For this review, use the dimensioned drawing (mm, ordinates from the lowest corner) and the shaded views. Give positions to 0.01 mm unless a question says otherwise; leave off trailing zeros. Order: outer loops, then holes, each group sorted by start corner. A loop starts at its lowest first (then second) coordinate and runs counter-clockwise, first axis right, second up.
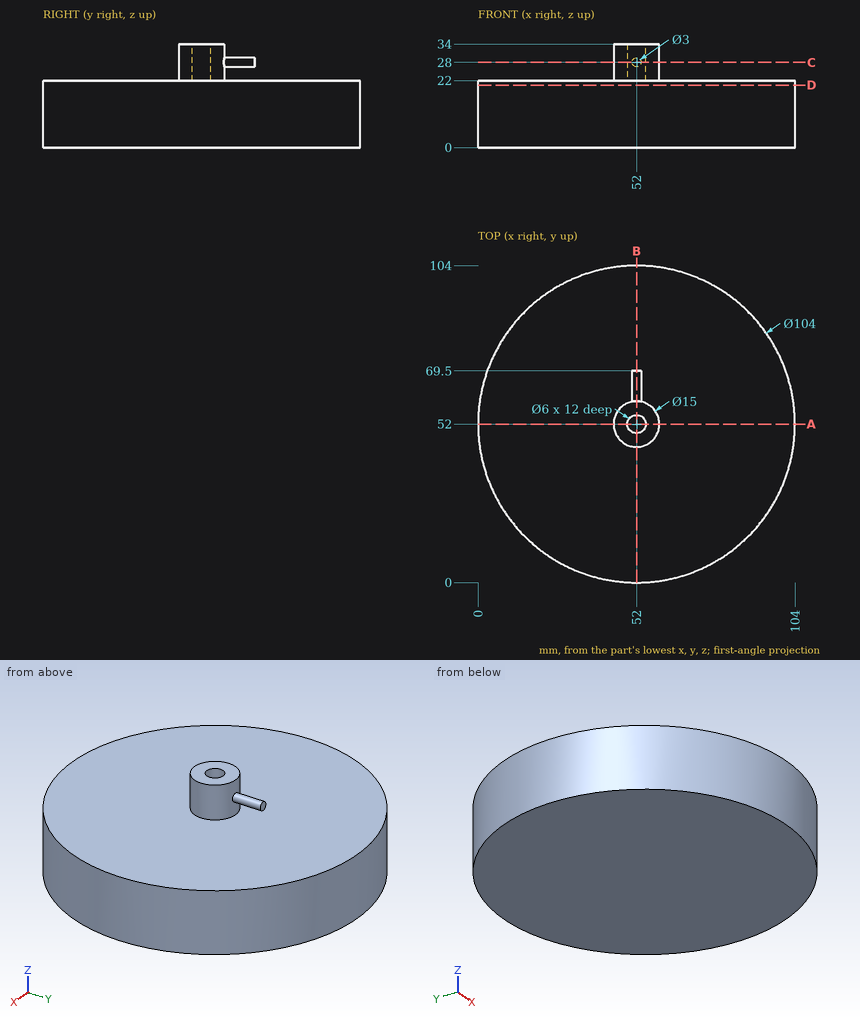
1. For line 1 along Y through (x, z) = (52, 24.5); line 2 along Z through (x, y) = (59.5, 58); line 3 along Y through (x, z) = (29, 17), list the stretches that pass through material, from the lowest coordinate up.
Recorded:
line 1: y = 44.5 to 49, 55 to 59.5
line 2: z = 0 to 22
line 3: y = 5.36 to 98.64
2. Take a section at B-B (x = 52). State the section outline as (y, z) points.
Recorded:
outline: (0, 0) - (104, 0) - (104, 22) - (59.5, 22) - (59.5, 26.5) - (69.5, 26.5) - (69.5, 29.5) - (59.5, 29.5) - (59.5, 34) - (55, 34) - (55, 22) - (49, 22) - (49, 34) - (44.5, 34) - (44.5, 22) - (0, 22) - close
3. Take a section at A-A (y = 52). State the section outline as (x, z) points.
Recorded:
outline: (0, 0) - (104, 0) - (104, 22) - (59.5, 22) - (59.5, 34) - (55, 34) - (55, 22) - (49, 22) - (49, 34) - (44.5, 34) - (44.5, 22) - (0, 22) - close
4. Take a section at C-C (z = 28). State the section outline as (x, y) points, then the cut area to 3 significant figures.
Recorded:
outline: (50.5, 59.35) arc R7.5 ccw (long way) to (53.5, 59.35) - (53.5, 69.5) - (50.5, 69.5) - close; hole circle Ø6 at (52, 52)
area: 179 mm2
5. For pin 1 (6 mm diameter, centred on y = 63.5, z = 19, fed in from +X); pin 2 (6 mm diameter, centred on y = 69, z = 8, fed in from +X); pin 3 (5 mm diameter, centred on x = 64.5, z = 11, fed in from +Y), all flat-tipped, find the tip position at first contact; note any pin that passes through.
Recorded:
pin 1: stops at x = 103.3
pin 2: stops at x = 102.08
pin 3: stops at y = 103.03
6. Take a section at D-D (z = 20.5). State the section outline as (x, y) points, then the cut area to 3 significant figures.
Recorded:
outline: circle Ø104 at (52, 52)
area: 8,490 mm2
